Autodesk Fusion 360 part; units mm, degrees
sketch "cadru" plane through (0, 0, 0) normal (1, 0, 0) x (0, 1, 0)
  line L0 (-20, -13.4697) -> (-20, 10.5303)
  line L1 (-17.5, -10.9697) -> (-17.5, 8.0303)
  line L2 (17.5, -10.9697) -> (-17.5, -10.9697)
  line L3 (20, -13.4697) -> (-20, -13.4697)
  line L4 (17.5, 8.0303) -> (17.5, -10.9697)
  line L5 (20, 10.5303) -> (20, -13.4697)
  line L6 (-20, 10.5303) -> (20, 10.5303)
  line L7 (-17.5, 8.0303) -> (17.5, 8.0303)
  line L8 (-1.25, 10.5303) -> (-1.25, 50.5303)
  line L9 (0, 0) -> (0, 50) construction
  line L10 (1.25, 10.5303) -> (1.25, 50.5303)
  line L11 (-1.25, 50.5303) -> (1.25, 50.5303)
  line L12 (17.5, -1.4697) -> (0, -1.4697) construction
  line L13 (-1.25, -53.4697) -> (1.25, -53.4697)
  line L14 (-1.25, -13.4697) -> (-1.25, -53.4697)
  line L15 (1.25, -13.4697) -> (1.25, -53.4697)
  line L16 (-20, -0.2197) -> (-70, -0.2197)
  line L17 (-70, -0.2197) -> (-70, -2.7197)
  line L18 (-70, -2.7197) -> (-20, -2.7197)
  line L19 (0, -1.4697) -> (-28.916, -1.4697) construction
  line L20 (-28.916, -1.4697) -> (-57.085, -1.4697) construction
  line L21 (-56.31, -0.6947) -> (-57.86, -0.6947)
  line L22 (-57.86, -0.6947) -> (-57.86, -2.2447)
  line L23 (-57.86, -2.2447) -> (-56.31, -2.2447)
  line L24 (-56.31, -2.2447) -> (-56.31, -0.6947)
  line L25 (-56.31, -0.6947) -> (-57.86, -2.2447) construction
  line L26 (-57.86, -0.6947) -> (-56.31, -2.2447) construction
  line L27 (-43.0005, -1.4697) -> (-43.0005, -15) construction
  line L28 (-45.0005, -5.2197) -> (-20, -5.2197)
  line L29 (-45.0005, -5.2197) -> (-45.0005, -0.2197)
  line L30 (-41.0005, -0.2197) -> (-41.0005, -5.2197)
  line L31 (-42.2255, -0.6947) -> (-43.7755, -0.6947)
  line L32 (-43.7755, -0.6947) -> (-43.7755, -2.2447)
  line L33 (-43.7755, -2.2447) -> (-42.2255, -2.2447)
  line L34 (-42.2255, -2.2447) -> (-42.2255, -0.6947)
  line L35 (-42.2255, -0.6947) -> (-43.7755, -2.2447) construction
  line L36 (-43.7755, -0.6947) -> (-42.2255, -2.2447) construction
  line L37 (-28.141, -0.6947) -> (-29.691, -0.6947)
  line L38 (-29.691, -0.6947) -> (-29.691, -2.2447)
  line L39 (-29.691, -2.2447) -> (-28.141, -2.2447)
  line L40 (-28.141, -2.2447) -> (-28.141, -0.6947)
  line L41 (-28.141, -0.6947) -> (-29.691, -2.2447) construction
  line L42 (-29.691, -0.6947) -> (-28.141, -2.2447) construction
  point P0 (-57.085, -1.4697)
  point P1 (-43.0005, -1.4697)
  point P2 (-28.916, -1.4697)
  dimension "d1" = -2.5
  dimension "d2" = 35
  dimension "d3" = 19
  dimension "d4" = 8.0303
  dimension "d5" = 17.5
  dimension "d6" = 40
  dimension "d7" = 1.25
  dimension "d10" = 50
  dimension "d11" = 2.5
  dimension "d12" = 1.25
  dimension "d13" = 28.916
  dimension "d15" = 28.169
  dimension "d16" = 1.55
  dimension "d17" = 1.55
  dimension "d22" = 14.0845
  dimension "d23" = 2.5
  dimension "d24" = 2
  dimension "d25" = 2
  dimension "d26" = 1.55
  dimension "d27" = 1.55
  dimension "d33" = 1.55
  dimension "d34" = 1.55
extrude "Extrude1" add sketch "cadru" along normal blind 5 contours L0 L3 L5 L6 | L0 L18 L28 L30 | L3 L13 L14 L15 | L0 L16 L18 L30 | L16 L18 L29 L30 | L16 L17 L18 L29 | L6 L8 L10 L11 | L31 L32 L33 L34
extrude "Extrude2" add sketch "cadru" along normal blind 15 contours L18 L28 L29 L30
extrude "Extrude3" add sketch "cadru" along normal blind 2.5 from surface at 15 contours L18 L28 L29 L30 | L16 L18 L29 L30
equation "d22 = ( 28.169 / 2 ) * 1 mm"
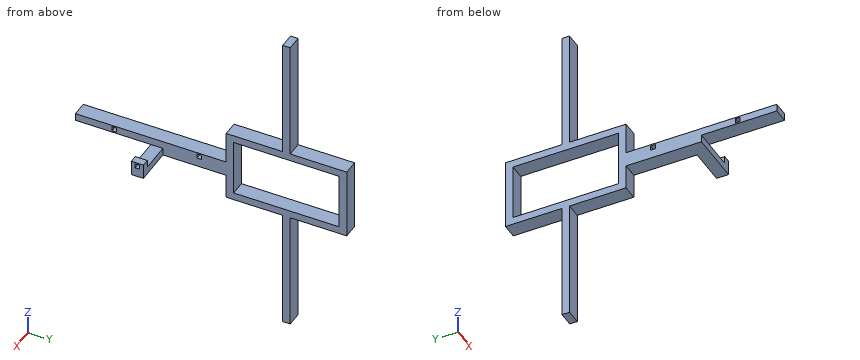
Check sheet for the modelled part. Datum: model origin and axes. Units: mm. Give positions to 0.01 mm unless a question says otherwise; leave off trailing zeros. Loops run counter-clockwise (first coordinate to the right, second up) from the corner with the lowest first, then second, coordinate; pieces in that order, holes last. Notation, with made-up numbers: M 3,2 L 55,2 A5 cw 55,9 Z; hole C -19.75,-16.5 d7. An arc over 180 degrees is marked long. Return JSON: item names as keys, results as strings. Group by question number.
1. Cross-section at D-D on y = -51. Record the boundary of the cut face in (x, z).
2. Cross-section at C-C on z = 26. Record the boundary of the cut face in (x, y).
3. Cross-section at A-A on y = -3.5. Record the boundary of the cut face in (x, z), plus the area to 3 significant figures.
4. Go/stop test with flat-tipped pins: pin 1 (0.5 mm diameter, centred on x = 16.5, z = -1.5, fed in from -Y); pin 2 (10 mm diameter, centred on x = 3, y = 10, fed in from -Z); pin 3 (5.5 mm diameter, centred on x = 3, z = 3.5, fed in from -Y). Record where each tip stops, or that it passes through.
5. Thickness scan on L1, parallel to Z at x = 1.5, y = 9; L2, parallel to Z at x = 3, y = -59.5; L3, parallel to Y at x = 3.75, z = 30. Record the ranges inside material, lowest first.
6. Cross-section at B-B on x = 16.25. Record the boundary of the cut face in (y, z).
Return value:
{
 "1": {"outline": "M 0,-2.72 L 5,-2.72 L 5,-0.22 L 0,-0.22 Z"},
 "2": {"outline": "M 0,-1.25 L 5,-1.25 L 5,1.25 L 0,1.25 Z"},
 "3": {"outline": "M 0,-13.47 L 5,-13.47 L 5,-10.97 L 0,-10.97 Z; M 0,8.03 L 5,8.03 L 5,10.53 L 0,10.53 Z", "area": "25.0 mm^2"},
 "4": {"pin 1": "y = -45", "pin 2": "z = -13.47", "pin 3": "y = -20"},
 "5": {"L1": "-13.47 to -10.97, 8.03 to 10.53", "L2": "-2.72 to -0.22", "L3": "-1.25 to 1.25"},
 "6": {"outline": "M -45,-5.22 L -41,-5.22 L -41,-0.22 L -45,-0.22 Z; hole M -43.78,-2.24 L -42.23,-2.24 L -42.23,-0.69 L -43.78,-0.69 Z"}
}
